```python
from build123d import *

# Parameters (mm, degrees)
SKETCH3_W           = 18.344
SKETCH3_H           = 6.63149511
BOSS_EXTRUDE2_DEPTH = 2.8


with BuildPart() as part:
    # Sketch3 → Boss-Extrude2 (new body)
    with BuildSketch(Plane.XY):
        with BuildLine():
            Line((55.495440626, -46.5265), (65.850440626, -46.5265))
            ThreePointArc((65.850440626, -46.5265), (72.921508438, -49.455432188), (75.850440626, -56.5265))
            Line((75.850440626, -56.5265), (75.850440626, -68.7965))
            Line((75.850440626, -68.7965), (82.058440626, -68.7965))
            Line((82.058440626, -68.7965), (82.058440626, -75.0055))
            Line((82.058440626, -75.0055), (75.850440626, -75.0055))
            Line((75.850440626, -75.0055), (75.850440626, -79.8025))
            Line((75.850440626, -79.8025), (70.486440626, -79.8025))
            Line((70.486440626, -79.8025), (70.486440626, -77.5455))
            Line((70.486440626, -77.5455), (66.818440626, -77.5455))
            Line((66.818440626, -77.5455), (66.818440626, -79.8025))
            Line((66.818440626, -79.8025), (62.020440626, -79.8025))
            Line((62.020440626, -79.8025), (62.020440626, -84.0365))
            Line((62.020440626, -84.0365), (66.818440626, -84.0365))
            Line((66.818440626, -84.0365), (66.818440626, -86.2935))
            Line((66.818440626, -86.2935), (70.486440626, -86.2935))
            Line((70.486440626, -86.2935), (70.486440626, -84.0365))
            Line((70.486440626, -84.0365), (75.850440626, -84.0365))
            Line((75.850440626, -84.0365), (75.850440626, -99.8395))
            Line((75.850440626, -99.8395), (82.058440626, -99.8395))
            Line((82.058440626, -99.8395), (82.058440626, -120.1605))
            Line((82.058440626, -120.1605), (75.850440626, -120.1605))
            Line((75.850440626, -120.1605), (75.850440626, -125.8055))
            Line((75.850440626, -125.8055), (70.486440626, -125.8055))
            Line((70.486440626, -125.8055), (70.486440626, -123.5475))
            Line((70.486440626, -123.5475), (66.818440626, -123.5475))
            Line((66.818440626, -123.5475), (66.818440626, -125.8055))
            Line((66.818440626, -125.8055), (62.020440626, -125.8055))
            Line((62.020440626, -125.8055), (62.020440626, -130.0385))
            Line((62.020440626, -130.0385), (66.818440626, -130.0385))
            Line((66.818440626, -130.0385), (66.818440626, -132.2955))
            Line((66.818440626, -132.2955), (70.486440626, -132.2955))
            Line((70.486440626, -132.2955), (70.486440626, -130.0385))
            Line((70.486440626, -130.0385), (75.850440626, -130.0385))
            Line((75.850440626, -130.0385), (75.850440626, -134.8365))
            Line((75.850440626, -134.8365), (82.058440626, -134.8365))
            Line((82.058440626, -134.8365), (82.058440626, -141.0445))
            Line((82.058440626, -141.0445), (75.850440626, -141.0445))
            Line((75.850440626, -141.0445), (75.850440626, -153.315747555))
            ThreePointArc((75.850440626, -153.315747555), (72.921508438, -160.386815367), (65.850440626, -163.315747555))
            Line((65.850440626, -163.315747555), (55.495440626, -163.315747555))
            ThreePointArc((55.495440626, -163.315747555), (48.424372815, -160.386815367), (45.495440626, -153.315747555))
            Line((45.495440626, -153.315747555), (45.495440626, -149.654747555))
            Line((45.495440626, -149.654747555), (45.495440626, -56.5265))
            ThreePointArc((45.495440626, -56.5265), (48.424372815, -49.455432188), (55.495440626, -46.5265))
        make_face()
        with Locations((60.71181161, -115.112247555)):
            Rectangle(SKETCH3_W, SKETCH3_H, mode=Mode.SUBTRACT)
    extrude(amount=BOSS_EXTRUDE2_DEPTH)


solid = part.part
```
CAD build for the part. Positions are in the model's coordinates, mm. A direction names the side the tool comes from. Round coordinates to 2 decimals unless told otherwise and drop trailing zeros. Write each loop counter-clockwise with the first axis right and the second up, starting at its lowest first coordinate (ties: lowest second). Pieces come first, ordered by that corner, then holes. Notation, with made-up numbers: (36.25, 26.25) -> (64.25, 26.25) arc R22 cw to (64.25, 39.25) -> close; hole circle Ø9 at (60.5, 11). An arc over 180 degrees is marked (long way). Answer in a Markdown table with one row per item. Add a question column.
Item 1: Saw through at D-D, the plane x = 49. Write the cut outline in (y, z).
Item 2: Saw through at C-C, the plane y = -91. Write the cut outline in (x, z), then the cut area to 3 significant figures.
Item 3: Drop flat-ended pins along their axis: pin 1 Ø1.4 at (y, z) = (-65.5, 2) entering from +X; pin 2 Ø1.4 at (x, z) = (80, 1.5) entering from -Y; pin 3 Ø1.4 at (x, z) = (69, 1.5) entering from +Y; pin 4 Ø1 at (x, y) = (50, -78) entering from -Z. Give the stop position or say it passes through.
Item 4: Saw through at B-B, the plane x = 71.5. Write the cut outline in (y, z).
Item 5: Saw through at A-A, the plane x = 63.5. Write the cut outline in (y, z), then the cut area to 3 significant figures.
Item 6: Which spindle directions (+Z, -Z, +X, -X, +Y, -Y) get a long thin tool onto all of the face, cutting with end or side? Do faces 1 (the face through (66.818, -131, 1)), 2 (the face through (64, -125.806, 1)), 3 (the face through (61, -163.316, 1)). Say none if no direction does.
Item 7: Mould opens along Y. For faces 4 (the face through (69, -86.294, 1)), 5 (the face through (48.5, -160.46, 1.38)), 6 (the face through (75.85, -147, 1)) say: pulls with the +Y half, pulls with the -Y half, needs draft (parallel to the pull), parting line crosses it, or undercut.
Item 8: Drill centre lines: line 1 (Y direction, x = 76, z = 1.2); line 2 (Y direction, x = 65.5, z = 0.2); line 3 (X direction, y = -124.5, z = 1.8). Where is each one in solid material? Low to high. Write a range as from..to.
Findings below:
| question | item | result |
|---|---|---|
| 1 | outline | (-160.92, 0) -> (-48.92, 0) -> (-48.92, 2.8) -> (-160.92, 2.8) -> close |
| 2 | outline | (45.5, 0) -> (75.85, 0) -> (75.85, 2.8) -> (45.5, 2.8) -> close |
| 2 | area | 85.0 mm^2 |
| 3 | pin 1 | stops at x = 75.85 |
| 3 | pin 2 | stops at y = -141.04 |
| 3 | pin 3 | stops at y = -46.83 |
| 3 | pin 4 | stops at z = 0 |
| 4 | outline | (-161.57, 0) -> (-130.04, 0) -> (-130.04, 2.8) -> (-161.57, 2.8) -> close; (-125.81, 0) -> (-84.04, 0) -> (-84.04, 2.8) -> (-125.81, 2.8) -> close; (-79.8, 0) -> (-48.28, 0) -> (-48.28, 2.8) -> (-79.8, 2.8) -> close |
| 5 | outline | (-163.32, 0) -> (-130.04, 0) -> (-130.04, 2.8) -> (-163.32, 2.8) -> close; (-125.81, 0) -> (-118.43, 0) -> (-118.43, 2.8) -> (-125.81, 2.8) -> close; (-111.8, 0) -> (-84.04, 0) -> (-84.04, 2.8) -> (-111.8, 2.8) -> close; (-79.8, 0) -> (-46.53, 0) -> (-46.53, 2.8) -> (-79.8, 2.8) -> close |
| 5 | area | 285 mm^2 |
| 6 | face 1 | +Z, -Z |
| 6 | face 2 | +Z, -Z, +X |
| 6 | face 3 | +Z, -Z, +X, -X, -Y |
| 7 | face 4 | undercut |
| 7 | face 5 | pulls with the -Y half |
| 7 | face 6 | needs draft |
| 8 | line 1 | y = -141.04..-134.84, -120.16..-99.84, -75.01..-68.8 |
| 8 | line 2 | y = -163.32..-130.04, -125.81..-118.43, -111.8..-84.04, -79.8..-46.53 |
| 8 | line 3 | x = 45.5..66.82, 70.49..75.85 |
